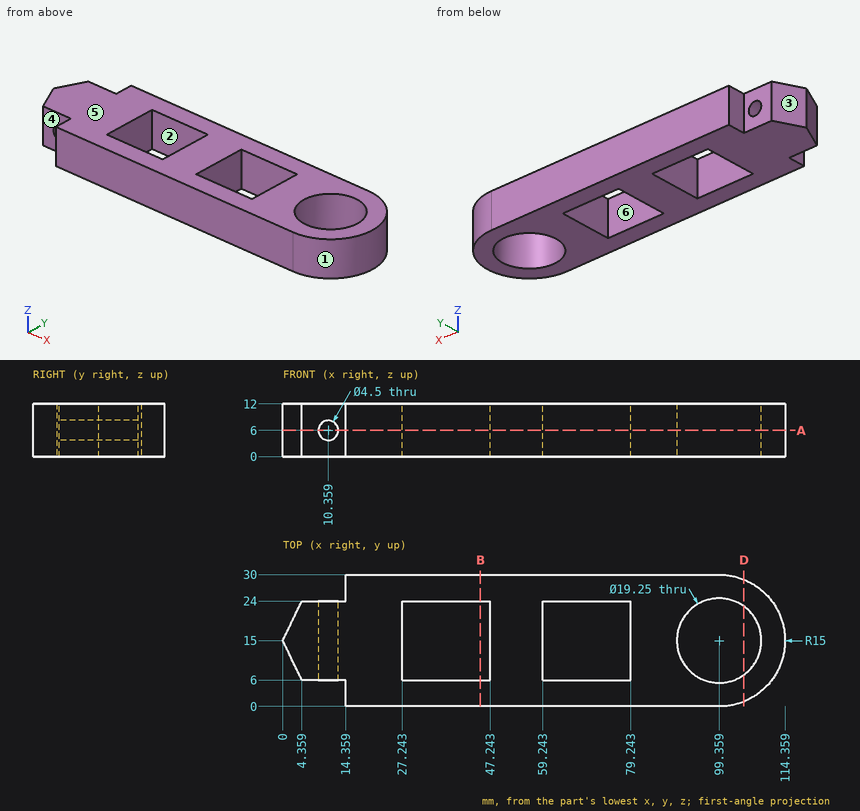
Design review of the part shown in the three views and the two pictorial views. Dimensions are in mm from the part's minimum x, y and z. A direction names the side the tool comes from. Round coordinates to 2 decimals unless told otherwise and drop trailing zeros. Loops run counter-clockwise (first coordinate to the right, second up) from the corner with the lowest first, then second, coordinate; pieces in that order, holes last. Notation, with made-up numbers: (-30, -16.75) -> (17, -16.75) arc R15 cw to (17, 12.25) -> close; hole circle Ø2 at (-6, 66). An arc over 180 degrees is marked (long way). Answer as a JSON object with one key per item and string values. Group by question number.
1) For pin 1 Ø3.5 at (y, z) = (12.5, 6.5) entering from -X; pin 2 Ø1.5 at (y, z) = (10, 6) entering from -X; pin 3 Ø3.5 at (y, z) = (13.5, 6) entering from -X; pin 4 Ø4 at (x, z) = (10.36, 6) entering from -Y, all flat-tipped, find the tip position at first contact; note any pin that passes through.
2) We need section D-D on x = 105. Write out the cut boundary in (y, z).
3) Mouldability with a two-part tool opening along Y and no side actions: class the marked faces 1, 2 and 3 as released by +Y, released by -Y, zero draft, split by the parting line, or undercut.
4) For line 1 (Y direction, x = 28, z = 6.25); line 2 (X direction, y = 13, z = 8) (1 decimal); line 3 (X direction, y = 8.75, z = 2.75) (1 decimal), list the stretches that pass through material, from the lowest coordinate up. Write a range as [from, to].
5) We need section B-B on x = 45. Write out the cut boundary in (y, z).
6) We need section A-A on z = 6. Give the number of separate pieces and of enclosed holes in the cut face, then the cut area to 3 significant figures.
7) For the marked faces 4, 5 and 6, list the 3-axis set-ups (+Z, -Z, +X, -X, +Y, -Y) from which the entire face can be reached by the end or side of a thin tool; tool diameter is ignored.
Result set:
{
 "1": {"pin 1": "x = 0.36", "pin 2": "x = 2.06", "pin 3": "x = 0", "pin 4": "through"},
 "2": {"outline": "(1.1, 0) -> (7.2, 0) -> (7.2, 12) -> (1.1, 12) -> close; (22.8, 0) -> (28.9, 0) -> (28.9, 12) -> (22.8, 12) -> close"},
 "3": {"face 1": "split by the parting line", "face 2": "undercut", "face 3": "released by +Y"},
 "4": {"line 1": "[0, 6], [24, 30]", "line 2": "[1, 9.3], [11.4, 27.2], [47.2, 59.2], [79.2, 89.9], [108.8, 114.2]", "line 3": "[3, 27.2], [47.2, 59.2], [79.2, 92], [106.7, 113]"},
 "5": {"outline": "(0, 0) -> (6, 0) -> (6, 12) -> (0, 12) -> close; (24, 0) -> (30, 0) -> (30, 12) -> (24, 12) -> close"},
 "6": {"separate pieces": "2", "enclosed holes": "3", "area": "2,030 mm²"},
 "7": {"face 4": "+Z, -Z, -X, -Y", "face 5": "+Z, +X, -X, +Y, -Y", "face 6": "+Z, -Z"}
}
